from build123d import *

# Parameters (mm, degrees)
SKETCH1_W           = 68
SKETCH1_H           = 150
BOSS_EXTRUDE1_DEPTH = 1
SKETCH2_R           = 2
CUT_EXTRUDE1_DEPTH  = 1
CUT_EXTRUDE2_DEPTH  = 20


with BuildPart() as part:
    # Sketch1 → Boss-Extrude1 (new body)
    with BuildSketch(Plane.XY):
        with Locations((34, 75)):
            Rectangle(SKETCH1_W, SKETCH1_H)
    extrude(amount=BOSS_EXTRUDE1_DEPTH)

    # Sketch2 → Cut-Extrude1 (cut)
    with BuildSketch(Plane.XY.offset(1)):
        with Locations((9.95, 14)):
            Circle(SKETCH2_R)
        with Locations((53, 14)):
            Circle(SKETCH2_R)
        with Locations(Location((53, 136, 0), (0, 0, 180))):
            Circle(SKETCH2_R)
        with Locations(Location((9.95, 136, 0), (0, 0, 180))):
            Circle(SKETCH2_R)
    extrude(amount=-CUT_EXTRUDE1_DEPTH, mode=Mode.SUBTRACT)

    # Sketch3 → Cut-Extrude2 (cut)
    with BuildSketch(Plane(origin=(0, 0, 0), x_dir=(-1, 0, 0), z_dir=(0, 0, -1))):
        Polygon((-35.78, 80.53), (-35.78, 123.74), (-55.64, 126.96), (-55.64, 83.01), align=None)
        Polygon((-55.64, 66.99), (-35.78, 69.47), (-35.78, 26.26), (-55.64, 23.04), align=None)
    extrude(amount=-CUT_EXTRUDE2_DEPTH, mode=Mode.SUBTRACT)


solid = part.part
Build history of the part. All positions in model axes, mm. A direction names the side the tool comes from. Give positions to 0.01 mm unless a question says otherwise; leave off trailing zeros. Order: outer loops, then holes, each group sorted by start corner. A loop starts at its lowest first (then second) coordinate and runs counter-clockwise, first axis right, second up. Notation, with made-up numbers: M -13.75,5.5 L 6.25,5.5 A25 ccw 6.25,38.5 Z; hole C -7,20.25 d10. An arc over 180 degrees is marked long. Put each result on its own line as item: value.
Item 1: Cut at A-A on y = 136. Write the cut outline in (x, z), then the cut area to 3 significant figures.
Results are:
outline: M 0,0 L 7.95,0 L 7.95,1 L 0,1 Z; M 11.95,0 L 51,0 L 51,1 L 11.95,1 Z; M 55,0 L 68,0 L 68,1 L 55,1 Z
area: 60.0 mm2
Item 2: Cut at D-D on x = 53. Write the cut outline in (y, z), then the cut area to 3 significant figures.
Results are:
outline: M 0,0 L 12,0 L 12,1 L 0,1 Z; M 16,0 L 23.47,0 L 23.47,1 L 16,1 Z; M 67.32,0 L 82.68,0 L 82.68,1 L 67.32,1 Z; M 126.53,0 L 134,0 L 134,1 L 126.53,1 Z; M 138,0 L 150,0 L 150,1 L 138,1 Z
area: 54.3 mm2
Item 3: Cut at C-C on y = 107. Write the cut outline in (x, z), then the cut area to 3 significant figures.
Results are:
outline: M 0,0 L 35.78,0 L 35.78,1 L 0,1 Z; M 55.64,0 L 68,0 L 68,1 L 55.64,1 Z
area: 48.1 mm2
Item 4: Wall check: probe 1 along Y at (x, z) = (9.95, 0.6); probe 2 along X at (y, z) = (111, 0.1); probe 3 along Y at (x, z) = (37, 0.3). Give the ranges that are in metal, low to high.
Results are:
probe 1: 0 to 12, 16 to 134, 138 to 150
probe 2: 0 to 35.78, 55.64 to 68
probe 3: 0 to 26.06, 69.32 to 80.68, 123.94 to 150
Item 5: Drop a flat-ended pin along its axis: pin 1 Ø3.5 at (x, y) = (53, 136) entering from -Z. Give the stop position or say it passes through.
Results are:
pin 1: through
Item 6: Cut at B-B on z = 0.55. Write the cut outline in (x, y), then the cut area to 3 significant figures.
Results are:
outline: M 0,0 L 68,0 L 68,150 L 0,150 Z; hole C 9.95,14 d4; hole C 9.95,136 d4; hole M 35.78,26.26 L 55.64,23.04 L 55.64,66.99 L 35.78,69.47 Z; hole M 35.78,80.53 L 55.64,83.01 L 55.64,126.96 L 35.78,123.74 Z; hole C 53,14 d4; hole C 53,136 d4
area: 8,420 mm2
Item 7: Which spindle directions (+Z, -Z, +X, -X, +Y, -Y) get a long thin tool onto all of the face, cutting with end or side? Do faces 3 (the face through (34, 76, 1)), 4 (the face through (45.571, 24.673, 0.493)). Say none if no direction does.
Results are:
face 3: +Z, +X, -X, +Y, -Y
face 4: +Z, -Z
Item 8: Pull direction X, two halves, no side cores. Call faces 1 (the face through (34, 76, 0)), 2 (the face through (45.849, 68.213, 0.493)): +X half, -X half, draft (parallel to the pull), parting line (faces both ways), or undercut.
Results are:
face 1: draft
face 2: undercut
